Build history of the part. All positions in model axes, mm. A direction names the side the tool comes from. Round coordinates to 2 decimals unless told otherwise and drop trailing zeros. Order: outer loops, then holes, each group sorted by start corner. A loop starts at its lowest first (then second) coordinate and runs counter-clockwise, first axis right, second up. Notation, with made-up numbers: (-2, -30) -> (56, -30) arc R17 ccw to (56, -14) -> close; hole circle Ø3 at (85.25, 77). An arc over 180 degrees is marked (long way). Write item = value, one per line.
from build123d import *

# Parameters (mm, degrees)
SKETCH1_R                         = 76.2
BOSS_EXTRUDE1_DEPTH               = 12.7
F_3_8_CLEARANCE_HOLE1_D           = 9.8044
F_1_4_CLEARANCE_HOLE1_D           = 6.5278
F_1_4_NPT_TAPPED_HOLE1_AT_2_COUNT = 2
F_1_4_NPT_TAPPED_HOLE1_AT_2_PITCH = 74.789953871
F_1_4_NPT_TAPPED_HOLE1_AT_3_COUNT = 2
F_1_4_NPT_TAPPED_HOLE1_AT_3_PITCH = 74.789953871
SKETCH8_R                         = 10.414
CUT_EXTRUDE1_DEPTH                = 109.508847566
CHAMFER1_SIZE                     = 3.175


with BuildPart() as part:
    # Sketch1 → Boss-Extrude1 (new body)
    with BuildSketch(Plane(origin=(0, 0, 0), x_dir=(1, 0, 0), z_dir=(0, 1, 0))):
        with Locations(Location((0, 0, 0), (0, 0, 270))):
            Circle(SKETCH1_R)
    extrude(amount=BOSS_EXTRUDE1_DEPTH)

    # 3/8 Clearance Hole1 (through all)
    with Locations(Plane(origin=(0, 12.7, 0), x_dir=(1, 0, 0), z_dir=(0, 1, 0))):
        with Locations((47.146344636, -47.146344636), (66.675, 0), (47.146344636, 47.146344636), (0, 66.675), (-47.146344636, 47.146344636), (-66.675, 0), (-47.146344636, -47.146344636), (0, -66.675)):
            Hole(F_3_8_CLEARANCE_HOLE1_D / 2)

    # 1/4 Clearance Hole1 (through all)
    with Locations(Plane(origin=(0, 12.7, 0), x_dir=(1, 0, 0), z_dir=(0, 1, 0))):
        with Locations((12.7, -21.997045256), (25.4, 0), (12.7, 21.997045256), (-12.7, 21.997045256), (-25.4, 0), (-12.7, -21.997045256)):
            Hole(F_1_4_CLEARANCE_HOLE1_D / 2)

    # Sketch7 → 1/4 NPT Tapped Hole1 (revolve, cut)
    with BuildSketch(Plane(origin=(-37.394976935, 12.7, -21.59), x_dir=(0, 0, 1), z_dir=(1, 0, 0))):
        Polygon((0, 0), (0, 12.7), (5.5626, 12.7), (5.5626, 9.906), (6.557984794, 9.906), (6.8545837, 0), align=None)
    f_1_4_npt_tapped_hole1 = revolve(axis=Axis((-37.394976935, 19.05, -21.59), (0, -1, 0)), mode=Mode.SUBTRACT)

    # 1/4 NPT Tapped Hole1 at 2: 1/4 NPT Tapped Hole1 ×2
    with Locations(*[Vector(0.5000000000000003, 0, 0.8660254037844386) * (i * F_1_4_NPT_TAPPED_HOLE1_AT_2_PITCH) for i in range(1, F_1_4_NPT_TAPPED_HOLE1_AT_2_COUNT)]):
        add(f_1_4_npt_tapped_hole1, mode=Mode.SUBTRACT)

    # 1/4 NPT Tapped Hole1 at 3: 1/4 NPT Tapped Hole1 ×2
    with Locations(*[(i * F_1_4_NPT_TAPPED_HOLE1_AT_3_PITCH, 0, 0) for i in range(1, F_1_4_NPT_TAPPED_HOLE1_AT_3_COUNT)]):
        add(f_1_4_npt_tapped_hole1, mode=Mode.SUBTRACT)

    # Sketch8 → Cut-Extrude1 (cut, through all)
    with BuildSketch(Plane(origin=(0, 12.7, 0), x_dir=(1, 0, 0), z_dir=(0, 1, 0))):
        with Locations(Location((0, 0, 0), (0, 0, 270))):
            Circle(SKETCH8_R)
    extrude(amount=-CUT_EXTRUDE1_DEPTH, mode=Mode.SUBTRACT)

    # Chamfer1
    chamfer1_edges = [part.edges().sort_by_distance(p)[0] for p in [
        (0, 12.7, -10.414),
    ]]
    chamfer(chamfer1_edges, length=CHAMFER1_SIZE)


solid = part.part
Q1. Cut at B-B, the plane x = 0. List the corners of the cut face in (y, z) (3 decimals), and give its area (3 significant figures).
Check values:
outline = (0, -76.2) -> (12.7, -76.2) -> (12.7, -71.577) -> (0, -71.577) -> close; (0, -61.773) -> (12.7, -61.773) -> (12.7, -13.589) -> (9.525, -10.414) -> (0, -10.414) -> close; (0, 10.414) -> (9.525, 10.414) -> (12.7, 13.589) -> (12.7, 36.325) -> (2.794, 36.622) -> (2.794, 37.617) -> (0, 37.617) -> close; (0, 48.743) -> (2.794, 48.743) -> (2.794, 49.738) -> (12.7, 50.035) -> (12.7, 61.773) -> (0, 61.773) -> close; (0, 71.577) -> (12.7, 71.577) -> (12.7, 76.2) -> (0, 76.2) -> close
area = 1,250 mm²
Q2. Which spindle directions (+Z, -Z, +X, -X, +Y, -Y) get a long thin tool onto all of the face, cutting with end or side? Do faces 1 (the face through (-44.046, 7.816, -22.463)), 2 (the face through (13.12, 6.26, 18.76)). Say none if no direction does.
Check values:
face_1 = +Y
face_2 = +Y, -Y
Q3. Probe probe 1 along X at (y, z) = (9.25, 21); probe 2 along X at (y, z) = (2.75, -19); probe 3 along X at (y, z) = (9.5, 48.5). List the from-to ranges inside material, lowest first.
Check values:
probe_1 = -73.25 to -15.81, -9.59 to 9.59, 15.81 to 73.25
probe_2 = -73.79 to -42.32, -32.47 to -13.99, -11.41 to 11.41, 13.99 to 32.47, 42.32 to 73.79
probe_3 = -58.77 to -51.86, -42.43 to -4.17, 4.17 to 42.43, 51.86 to 58.77
Q4. Mould opens along Z. For faces 3 (the face through (-2.635, 6.261, -70.809)), 4 (the face through (-46.367, 6.261, -60.47)), 5 (the face through (-16, 0, -1)), 6 (the face through (-41.154, 1.417, -25.69)) say: released by +Z, released by -Z, zero draft, split by the parting line, or undercut.
Check values:
face_3 = undercut
face_4 = split by the parting line
face_5 = zero draft
face_6 = undercut
Q5. Flat gauge pins, fed straight in: pin 1 (11.5 mm diameter, centred on x = 47.15, z = 47.15, fed in from +Y); pin 2 (13 mm diameter, centred on x = -37.39, z = -21.59, fed in from +Y); pin 3 (3 mm diameter, centred on y = 2, z = -1, fed in from -X); pin 4 (1.5 mm diameter, centred on x = -31.5, y = 6.5, fed in from -Z). Where does each tip first touch, or does it go through?
Check values:
pin_1 = 12.7
pin_2 = 2.79
pin_3 = -76.2
pin_4 = -69.72
Q6. Cut at A-A, the plane z = 0. List the corners of the cut face in (x, y) (3 decimals).
Check values:
outline = (-76.2, 0) -> (-71.577, 0) -> (-71.577, 12.7) -> (-76.2, 12.7) -> close; (-61.773, 0) -> (-28.664, 0) -> (-28.664, 12.7) -> (-61.773, 12.7) -> close; (-22.136, 0) -> (-10.414, 0) -> (-10.414, 9.525) -> (-13.589, 12.7) -> (-22.136, 12.7) -> close; (10.414, 0) -> (22.136, 0) -> (22.136, 12.7) -> (13.589, 12.7) -> (10.414, 9.525) -> close; (28.664, 0) -> (61.773, 0) -> (61.773, 12.7) -> (28.664, 12.7) -> close; (71.577, 0) -> (76.2, 0) -> (76.2, 12.7) -> (71.577, 12.7) -> close
Q7. Cut at C-C, the plane x = 25.4. List the corners of the cut face in (y, z).
Check values:
outline = (0, -71.84) -> (12.7, -71.84) -> (12.7, -3.26) -> (0, -3.26) -> close; (0, 3.26) -> (12.7, 3.26) -> (12.7, 71.84) -> (0, 71.84) -> close
Q8. Cut at D-D, the plane z = 64.5. List the corners of the cut face in (x, y), and give its area (3 significant figures).
Check values:
outline = (-40.57, 0) -> (-4.39, 0) -> (-4.39, 12.7) -> (-40.57, 12.7) -> close; (4.39, 0) -> (40.57, 0) -> (40.57, 12.7) -> (4.39, 12.7) -> close
area = 919 mm²
